The listing builds one solid part. Answer for the finished solid, in the listing's coordinates (mm). Face numbers are marked on the shaded views. A direction names the side the tool comes from. Round coordinates to 2 decimals unless told otherwise and drop trailing zeros. Write each loop counter-clockwise with the first axis right and the second up, starting at its lowest first coordinate (ties: lowest second). Pieces come first, ordered by that corner, then holes.
Item 1: Find section A-A on x = 0. Give the vertices of the cut face in (y, z), then the cut area to 3 significant figures.
Item 2: Find section C-C on x = -14. Give the vertices of the cut face in (y, z).
Item 3: Find section D-D on x = -6.5. Give the vertices of the cut face in (y, z).
Item 4: A tool of negligible diameter and unlimited length cuts with its end or side. For the marked faces 1, 2 and 3, from which of +Z, -Z, +X, -X, +Y, -Y can it reach the whole face along a straight path? Write none if from no direction.
Item 5: Find the intervals of material crossed by probe 1 along Z at (x, y) = (0, -14); probe 2 along X at (y, z) = (-27, 10.2); probe 3 along Z at (x, y) = (-10.5, -16.5), in increasing order.
Item 6: Find section B-B on y = -15.5. Give the vertices of the cut face in (x, z), then the cut area to 3 significant figures.
Item 7: Each of these flat-tipped pins is pushed along its axis until it touches: pin 1 (4 mm diameter, centred on y = -17.5, z = 6.5, fed in from -X); pin 2 (5 mm diameter, centred on x = 12, y = -17, fed in from +Z); pin 3 (0.8 mm diameter, centred on y = -27.5, z = 9.5, fed in from +X). Where does it stop, or does it pass through?
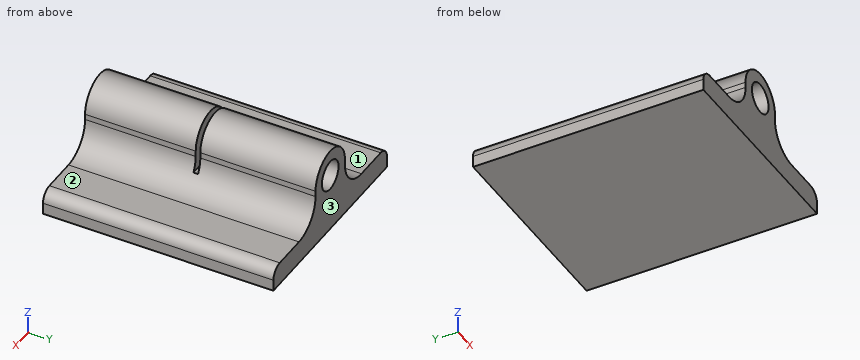
```python
from build123d import *

# Parameters (mm, degrees)
F0_R     = 2.6
F1_DEPTH = 40
F2_W     = 0.8
F2_H     = 8.2
F3_DEPTH = 35.601
F4_R     = 2


with BuildPart() as f1:
    # F0 (on Front) → F1 (new body)
    with BuildSketch(Plane.XZ):
        with BuildLine():
            Line((-17.8, 4), (-17.8, 0))
            Line((-17.8, 0), (17.8, 0))
            Line((17.8, 0), (17.8, 4))
            Line((17.8, 4), (9.8, 4))
            ThreePointArc((9.8, 4), (6.123045, 5.523045), (4.6, 9.2))
            Line((4.6, 9.2), (4.6, 10.2))
            ThreePointArc((4.6, 10.2), (0, 14.8), (-4.6, 10.2))
            Line((-4.6, 10.2), (-4.6, 9.2))
            ThreePointArc((-4.6, 9.2), (-6.123045, 5.523045), (-9.8, 4))
            Line((-9.8, 4), (-17.8, 4))
        make_face()
        with Locations((0, 10.2)):
            Circle(F0_R, mode=Mode.SUBTRACT)
    extrude(amount=F1_DEPTH)

    # F2 (on face) → F3 (cut, through all)
    with BuildSketch(Plane.YZ.offset(17.8)):
        with Locations((-20.4, 10.7)):
            Rectangle(F2_W, F2_H)
    extrude(amount=-F3_DEPTH, mode=Mode.SUBTRACT)

    # F4
    f4_edges = [f1.edges().sort_by_distance(p)[0] for p in [
        (-17.8, -20, 4),
        (17.8, -20, 4),
    ]]
    fillet(f4_edges, radius=F4_R)


solid = f1.part
```
Check values:
1. outline: (-40, 0) - (0, 0) - (0, 7.6) - (-20, 7.6) - (-20, 6.6) - (-20.8, 6.6) - (-20.8, 7.6) - (-40, 7.6) - close; (-40, 12.8) - (-20.8, 12.8) - (-20.8, 14.8) - (-40, 14.8) - close; (-20, 12.8) - (0, 12.8) - (0, 14.8) - (-20, 14.8) - close
1. area: 382 mm2
2. outline: (-40, 0) - (0, 0) - (0, 4) - (-40, 4) - close
3. outline: (-40, 0) - (0, 0) - (0, 5.18) - (-40, 5.18) - close
4. face 1: +Z, -X, +Y, -Y
4. face 2: +Z, +X, +Y, -Y
4. face 3: +Z, -Z, +X, -X, +Y
5. probe 1: z = 0 to 7.6, 12.8 to 14.8
5. probe 2: x = -4.6 to -2.6, 2.6 to 4.6
5. probe 3: z = 0 to 4
6. outline: (-17.8, 0) - (17.8, 0) - (17.8, 2) arc R2 ccw to (15.8, 4) - (9.8, 4) arc R5.2 cw to (4.6, 9.2) - (4.6, 10.2) arc R4.6 ccw to (-4.6, 10.2) - (-4.6, 9.2) arc R5.2 cw to (-9.8, 4) - (-15.8, 4) arc R2 ccw to (-17.8, 2) - close; hole circle Ø5.2 at (0, 10.2)
6. area: 221 mm2
7. pin 1: stops at x = -7.58
7. pin 2: stops at z = 4.01
7. pin 3: stops at x = 4.6
